Geometry check sheet. Reference: the model listing, model coordinates, mm. Face numbers are marked on the shaded views. Round coordinates to 2 decimals unless told otherwise and drop trailing zeros. Write each loop counter-clockwise with the first axis right and the second up, starting at its lowest first coordinate (ties: lowest second). Pieces come first, ordered by that corner, then holes.
Item 1: Scan lines: probe 1 along Y at (x, z) = (0, 18); probe 2 along Y at (x, z) = (-14, 11.5); probe 3 along Z at (x, y) = (-40.5, -6). Record each from-to range of solid material in increasing order.
Item 2: Cross-section at B-B (y = 53). Enter the section's corners in (x, z).
Item 3: Cross-section at D-D (y = 0). Enter the section's corners in (x, z), then the cut area to 3 significant figures.
Item 4: Cross-section at A-A (x = 0). Enter the section's corners in (y, z).
Item 5: Draft check along Y on the marked faces 1, 2, 3 and 4. Enter one of: pulls with the +Y half, pulls with the -Y half, needs draft (parallel to the pull), parting line crosses it, or undercut.
Item 6: Depth check by flat-ended pin: P1, Ø12, axis at x = 25, z = 33, coming from the -Y side; P2, Ø2, axis at y = -43, z = 29.5, coming from the +X side; P3, Ø18.5, axis at x = -13.5, y = 0.5, coming from the +Z side; P4, Ø1.5, axis at x = -40.5, z = 30, coming from the +Y side. Enter the tip coordinate at first touch or a pass-through.
Item 7: Cross-section at C-C (z = 4.5). Enter the section's corners in (x, y).
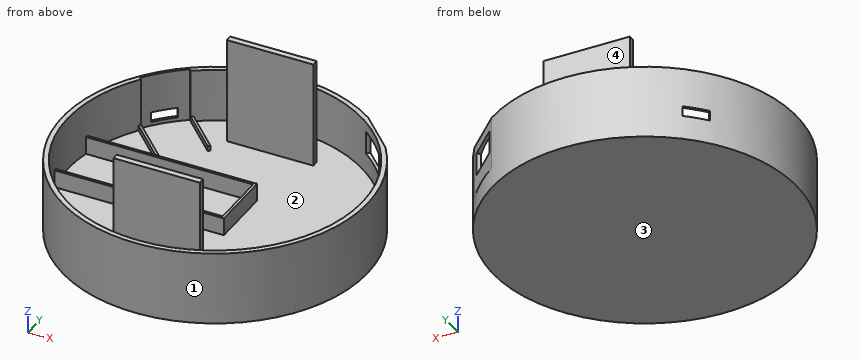
from build123d import *

# Parameters (mm, degrees)
CROQUIS1_R              = 60
SALIENTE_EXTRUIR1_DEPTH = 8
SALIENTE_EXTRUIR2_DEPTH = 7
CROQUIS3_R              = 60
CROQUIS3_R_2            = 58
SALIENTE_EXTRUIR3_DEPTH = 21
SALIENTE_EXTRUIR4_DEPTH = 2
CORTAR_EXTRUIR1_DEPTH   = 88.412813706
CORTAR_EXTRUIR2_START   = 1.5
CORTAR_EXTRUIR2_DEPTH   = 4
CORTAR_EXTRUIR3_DEPTH   = 88.412813706
CROQUIS9_W              = 9
CROQUIS9_H              = 15
CORTAR_EXTRUIR4_DEPTH   = 4
CROQUIS4_W              = 34
CROQUIS4_H              = 2.5
SALIENTE_EXTRUIR5_DEPTH = 42


with BuildPart() as part:
    # Croquis1 → Saliente-Extruir1 (new body)
    with BuildSketch(Plane.XY):
        Circle(CROQUIS1_R)
    extrude(amount=SALIENTE_EXTRUIR1_DEPTH)

    # Croquis2 → Saliente-Extruir2 (add)
    with BuildSketch(Plane.XY.offset(8)):
        Polygon((-56, 11.5), (9, 11.5), (9, -11.5), (-56, -11.5), (-57, -11.5), (-57, -12.5), (10, -12.5), (10, 12.5), (-57, 12.5), (-57, 11.5), align=None)
    extrude(amount=SALIENTE_EXTRUIR2_DEPTH)

    # Croquis3 → Saliente-Extruir3 (add)
    with BuildSketch(Plane.XY.offset(8)):
        Circle(CROQUIS3_R)
        with Locations(Location((0, 0, 0), (0, 0, 168.56384578))):
            Circle(CROQUIS3_R_2, mode=Mode.SUBTRACT)
    extrude(amount=SALIENTE_EXTRUIR3_DEPTH)

    # Croquis5 → Saliente-Extruir4 (add)
    with BuildSketch(Plane.XY.offset(8)):
        with BuildLine():
            Line((-19.984781547, 32.755130015), (-34.126917171, 46.897265639))
            ThreePointArc((-34.126917171, 46.897265639), (-41.012193309, 41.012193309), (-46.897265639, 34.126917171))
            Line((-46.897265639, 34.126917171), (-32.755130015, 19.984781547))
            Line((-32.755130015, 19.984781547), (-33.462236796, 19.277674766))
            Line((-33.462236796, 19.277674766), (-48.204317574, 34.019755543))
            ThreePointArc((-48.204317574, 34.019755543), (-41.71930009, 41.71930009), (-34.019755543, 48.204317574))
            Line((-34.019755543, 48.204317574), (-19.277674766, 33.462236796))
            Line((-19.277674766, 33.462236796), (-19.984781547, 32.755130015))
        make_face()
    extrude(amount=SALIENTE_EXTRUIR4_DEPTH)

    # Croquis6 → Cortar-Extruir1 (cut, through all)
    with BuildSketch(Plane.XY.offset(8)):
        with BuildLine():
            Line((-47.705839185, 34.715312294), (-46.897265639, 34.126917171))
            ThreePointArc((-46.897265639, 34.126917171), (-41.012193309, 41.012193309), (-34.126917171, 46.897265639))
            Line((-34.126917171, 46.897265639), (-34.715312294, 47.705839185))
            ThreePointArc((-34.715312294, 47.705839185), (-41.71930009, 41.71930009), (-47.705839185, 34.715312294))
        make_face()
    extrude(amount=CORTAR_EXTRUIR1_DEPTH, mode=Mode.SUBTRACT)

    # Croquis7 → Cortar-Extruir2 (cut)
    with BuildSketch(Plane.XY.offset(8).offset(CORTAR_EXTRUIR2_START)):
        Polygon((-35.355339059, 42.426406871), (-42.426406871, 49.497474683), (-49.497474683, 42.426406871), (-42.426406871, 35.355339059), align=None)
    extrude(amount=CORTAR_EXTRUIR2_DEPTH, mode=Mode.SUBTRACT)

    # Croquis8 → Cortar-Extruir3 (cut, through all)
    with BuildSketch(Plane.XY.offset(8)):
        with BuildLine():
            Line((48.904069139, 34.761933515), (34.761933515, 48.904069139))
            ThreePointArc((34.761933515, 48.904069139), (42.426406871, 42.426406871), (48.904069139, 34.761933515))
        make_face()
    extrude(amount=CORTAR_EXTRUIR3_DEPTH, mode=Mode.SUBTRACT)

    # Croquis9 → Cortar-Extruir4 (cut)
    with BuildSketch(Plane(origin=(41.833001327, 41.833001327, 0), x_dir=(0, 0, -1), z_dir=(0.7071067811865464, 0.7071067811865488, 0))):
        with Locations((-20.5, 0)):
            Rectangle(CROQUIS9_W, CROQUIS9_H)
    extrude(amount=-CORTAR_EXTRUIR4_DEPTH, mode=Mode.SUBTRACT)

    # Croquis4 → Saliente-Extruir5 (add)
    with BuildSketch(Plane.XY.offset(8)):
        with Locations((0, 42.75)):
            Rectangle(CROQUIS4_W, CROQUIS4_H)
        with Locations((0, -42.75)):
            Rectangle(CROQUIS4_W, CROQUIS4_H)
    extrude(amount=SALIENTE_EXTRUIR5_DEPTH)


solid = part.part
Resolved:
1. probe 1: y = -60 to -58, -44 to -41.5, 41.5 to 44, 58 to 60
1. probe 2: y = -58.34 to -56.28, -44 to -41.5, -12.5 to -11.5, 11.5 to 12.5, 41.5 to 44, 56.28 to 58.34
1. probe 3: z = 0 to 8
2. outline: (-28.12, 0) - (28.12, 0) - (28.12, 29) - (23.56, 29) - (23.56, 8) - (-23.56, 8) - (-23.56, 29) - (-28.12, 29) - close
3. outline: (-60, 0) - (60, 0) - (60, 29) - (58, 29) - (58, 8) - (10, 8) - (10, 15) - (9, 15) - (9, 8) - (-58, 8) - (-58, 29) - (-60, 29) - close
3. area: 1,050 mm2
4. outline: (-60, 0) - (60, 0) - (60, 29) - (58, 29) - (58, 8) - (44, 8) - (44, 50) - (41.5, 50) - (41.5, 8) - (12.5, 8) - (12.5, 15) - (11.5, 15) - (11.5, 8) - (-11.5, 8) - (-11.5, 15) - (-12.5, 15) - (-12.5, 8) - (-41.5, 8) - (-41.5, 50) - (-44, 50) - (-44, 8) - (-58, 8) - (-58, 29) - (-60, 29) - close
5. face 1: parting line crosses it
5. face 2: undercut
5. face 3: needs draft
5. face 4: undercut
6. P1: stops at y = -56.38
6. P2: stops at x = 42.72
6. P3: stops at z = 8
6. P4: passes through
7. outline: circle Ø120 at (0, 0)
